Read the model definition and answer for the solid it produces. Units are mm, in the model's axes. Face numbers are marked on the shaded views. Coordinates: 2 decimals unless noted, no trailing zeros. Loops run counter-clockwise (first coordinate to the right, second up) from the corner with the lowest first, then second, coordinate; pieces in that order, holes last. Notation, with made-up numbers: (35.25, 8.5) -> (61.25, 8.5) arc R24 cw to (61.25, 37.5) -> close; hole circle Ø3 at (55, 67). An arc over 180 degrees is marked (long way). Answer in a Markdown table with one row per item.
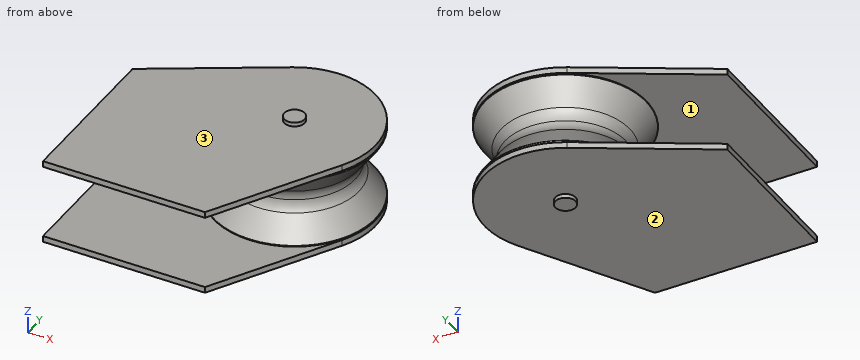
```python
from build123d import *
from build123d import SkipClean  # not in build123d's __all__

# Parameters (mm, degrees)
F0_W     = 25
F0_H     = 10
F0_H_2   = 15
F0_W_2   = 175
F5_DEPTH = 15


# Not quite as in the source:
# - ends of sketch curves that miss each other by under 0.0002 mm in the source are joined


with BuildPart() as f1:
    # F0 (on Right) → F1 (revolve)
    with BuildSketch(Plane.YZ):
        with Locations((12.5, 111)):
            Rectangle(F0_W, F0_H)
        with Locations((12.5, 98.5)):
            Rectangle(F0_W, F0_H_2)
        Polygon((0, 0), (25, 0), (25, 90), (25, 91), (0, 91), align=None)
    revolve(axis=Axis((0, 0, 58), (0, 0, 1)))

    # F0 (on Right) → F2 (revolve)
    with BuildSketch(Plane.YZ):
        with BuildLine():
            ThreePointArc((150, 0), (152.3425507406, 15.1250629778), (159.1507012033, 28.8328768565))
            Line((159.1507012033, 28.8328768565), (199.542465, 86.058356))
            ThreePointArc((199.542465, 86.058356), (199.7196970287, 88.6501935058), (197.5, 90))
            Line((197.5, 90), (25, 90))
            Line((25, 90), (25, 0))
            Line((25, 0), (150, 0))
        make_face()
    revolve(axis=Axis((0, 0, 58), (0, 0, 1)))

    # F0 (on Right) → F3 (revolve)
    with BuildSketch(Plane.YZ):
        with Locations((112.5, 98.5)):
            Rectangle(F0_W_2, F0_H_2)
    revolve(axis=Axis((0, 0, 58), (0, 0, 1)))

    # F4 (on face) → F5 (join, through all)
    with BuildSketch(Plane.XY.offset(106)):
        with BuildLine():
            ThreePointArc((0, -200), (-141.4213562373, -141.4213562373), (-200, 0))
            Line((-200, 0), (-400, 0))
            Line((-400, 0), (-400, -400))
            Line((-400, -400), (0, -400))
            Line((0, -400), (0, -200))
        make_face()
        with BuildLine():
            Line((-400, 0), (-200, 0))
            ThreePointArc((-200, 0), (-173.2050807569, 100), (-100, 173.2050807569))
            Line((-100, 173.2050807569), (-400, 0))
        make_face()
        with BuildLine():
            ThreePointArc((173.2050807569, -100), (100, -173.2050807569), (0, -200))
            Line((0, -200), (0, -400))
            Line((0, -400), (173.2050807569, -100))
        make_face()
    extrude(amount=-F5_DEPTH)

    # F6: F1 across face


with BuildPart() as f1_1:
    add(f1.part, clean=False)
    with SkipClean():  # cleaning this boolean's faces spoils the solid; the shape is the same uncleaned
        add(f1.part.mirror(Plane(origin=(0, 0, 0), x_dir=(1, 0, 0), z_dir=(0, 0, -1))), clean=False)


solid = f1_1.part
```
1. A cutting plane is placed at A-A on x = -342.5. Give the vertices of the cut face in (y, z).
A:
| item | result |
|---|---|
| outline | (-400, -106) -> (33.2, -106) -> (33.2, -91) -> (-400, -91) -> close; (-400, 91) -> (33.2, 91) -> (33.2, 106) -> (-400, 106) -> close |
2. The mould has two halves that part along Z. Classify the marked faces 1, 2 and 3: pulls with the +Z half, pulls with the -Z half, needs draft (parallel to the pull), parting line crosses it, or undercut.
A:
| item | result |
|---|---|
| face 1 | undercut |
| face 2 | pulls with the -Z half |
| face 3 | pulls with the +Z half |
3. Given pin 1 Ø1 at (x, y) = (-0.5, -250.5) entering from -Z; pin 2 Ø12 at (x, y) = (11, 32) entering from +Z; pin 3 Ø1 at (y, z) = (-68.5, 78.5) entering from +X, each flat-ended and moving along its own axis, determine where each tip first touches the part or whether it passes through.
A:
| item | result |
|---|---|
| pin 1 | stops at z = -106 |
| pin 2 | stops at z = 106 |
| pin 3 | stops at x = 182.15 |
4. A cutting plane is placed at C-C on y = 139. Count the separate pieces of the cut face and the enclosed holes in it, and give its area (3 significant figures).
A:
| item | result |
|---|---|
| separate pieces | 3 |
| enclosed holes | 0 |
| area | 44,400 mm2 |
5. Find the intervals of material crossed by probe 1 along Z at (x, y) = (82.5, -64); probe 2 along Z at (x, y) = (-297.5, -196); probe 3 along Y at (x, z) = (26, -34), in increasing order.
A:
| item | result |
|---|---|
| probe 1 | z = -106 to -91, -90 to 90, 91 to 106 |
| probe 2 | z = -106 to -91, 91 to 106 |
| probe 3 | y = -160.71 to 160.71 |
6. A cutting plane is placed at B-B on y = -294. Give the vertices of the cut face in (x, z), and give its area (3 significant figures).
A:
| item | result |
|---|---|
| outline | (-400, -106) -> (61.2, -106) -> (61.2, -91) -> (-400, -91) -> close; (-400, 91) -> (61.2, 91) -> (61.2, 106) -> (-400, 106) -> close |
| area | 13,800 mm2 |
